from build123d import *

# Parameters (mm, degrees)
SKETCH3_R           = 1.25
BOSS_EXTRUDE1_DEPTH = 3
FILLET1_R           = 0.75
FILLET2_R           = 1


with BuildPart() as part:
    # Sketch3 → Boss-Extrude1 (new body)
    with BuildSketch(Plane(origin=(0, 0, 0), x_dir=(1, 0, 0), z_dir=(0, 1, 0))):
        with BuildLine():
            Line((-11.5, -24), (-11.5, -27))
            Line((-11.5, -27), (11.5, -27))
            Line((11.5, -27), (11.5, -24))
            Line((11.5, -24), (12.25, -24))
            ThreePointArc((12.25, -24), (15.25, -21), (12.25, -18))
            Line((12.25, -18), (11.5, -18))
            Line((11.5, -18), (11.5, -6))
            Line((11.5, -6), (12.25, -6))
            ThreePointArc((12.25, -6), (15.25, -3), (12.25, 0))
            Line((12.25, 0), (-12.25, 0))
            ThreePointArc((-12.25, 0), (-15.25, -3), (-12.25, -6))
            Line((-12.25, -6), (-11.5, -6))
            Line((-11.5, -6), (-11.5, -18))
            Line((-11.5, -18), (-12.25, -18))
            ThreePointArc((-12.25, -18), (-15.25, -21), (-12.25, -24))
            Line((-12.25, -24), (-11.5, -24))
        make_face()
        with Locations(Location((-12.25, -21, 0), (0, 0, 90))):
            Circle(SKETCH3_R, mode=Mode.SUBTRACT)
        with Locations(Location((-12.25, -3, 0), (0, 0, 90))):
            Circle(SKETCH3_R, mode=Mode.SUBTRACT)
        with Locations(Location((12.25, -3, 0), (0, 0, 270))):
            Circle(SKETCH3_R, mode=Mode.SUBTRACT)
        with Locations(Location((12.25, -21, 0), (0, 0, 270))):
            Circle(SKETCH3_R, mode=Mode.SUBTRACT)
    extrude(amount=BOSS_EXTRUDE1_DEPTH)

    # Fillet1
    fillet1_edges = [part.edges().sort_by_distance(p)[0] for p in [
        (-11.5, 1.5, 18),
        (-11.5, 1.5, 24),
        (-11.5, 1.5, 6),
        (11.5, 1.5, 6),
        (11.5, 1.5, 24),
        (11.5, 1.5, 18),
    ]]
    fillet(fillet1_edges, radius=FILLET1_R - 0.0001)  # a hair under: the kernel refuses the full size

    # Fillet2
    fillet2_edges = [part.edges().sort_by_distance(p)[0] for p in [
        (15.25, 3, 21),
        (15.25, 3, 3),
        (0, 3, 0),
        (-15.25, 3, 3),
        (-15.25, 3, 21),
        (-11.5, 3, 12),
        (-11.5, 3, 25.87495),
        (11.5, 3, 12),
        (-11.719640625, 3, 17.780359375),
        (-11.719640625, 3, 24.219640625),
        (-11.719640625, 3, 6.219640625),
        (11.719640625, 3, 6.219640625),
        (11.719640625, 3, 24.219640625),
        (11.719640625, 3, 17.780359375),
        (11.5, 3, 25.87495),
    ]]
    fillet(fillet2_edges, radius=FILLET2_R)


solid = part.part
Part model, mm, in its own coordinate system. A direction names the side the tool comes from. Give positions to 0.01 mm unless a question says otherwise; leave off trailing zeros. Order: outer loops, then holes, each group sorted by start corner. A loop starts at its lowest first (then second) coordinate and runs counter-clockwise, first axis right, second up. Notation, with made-up numbers: (40.25, 67) -> (76.25, 67) arc R6 cw to (76.25, 73) -> close; hole circle Ø10 at (18.5, 32.5). An arc over 180 degrees is marked (long way). Use one line per item in the form item = value.
(1) Saw through at A-A (z = 3). Write the cut outline in (x, y).
Solution:
outline = (-15.25, 0) -> (-13.5, 0) -> (-13.5, 3) -> (-14.25, 3) arc R1 ccw to (-15.25, 2) -> close; (-11, 0) -> (11, 0) -> (11, 3) -> (-11, 3) -> close; (13.5, 0) -> (15.25, 0) -> (15.25, 2) arc R1 ccw to (14.25, 3) -> (13.5, 3) -> close
(2) Pull direction Z, two halves, no side cores. Call faces 4 (the face through (13, 1, 22)), 5 (the face through (11.5, 1, 26)), 6 (the face through (0, 1, 27)), 7 (the face through (11.5, 1, 12)): +Z half, -Z half, draft (parallel to the pull), parting line (faces both ways), or undercut.
Solution:
face_4 = undercut
face_5 = draft
face_6 = +Z half
face_7 = undercut
(3) Tool access for faces 1 (the face through (11.199, 2.715, 25.859)), 2 (the face through (15.25, 0.99, 3.07)), 3 (the face through (-11.199, 2.715, 25.891)): list every direction of +Z, -Z, +X, -X, +Y, -Y with a clear straight run to the whole face (end or side of a thin tool).
Solution:
face_1 = +Z, +X, +Y
face_2 = +X, +Y, -Y
face_3 = +Z, -X, +Y
(4) Flat gauge pins, fed straight in: P1, Ø1.6, axis at y = 0.5, z = 13.5, coming from the +X side; P2, Ø1.5, axis at x = 1, z = 17, coming from the -Y side; P3, Ø1, axis at y = 1, z = 26, coming from the -X side; P4, Ø1.5, axis at x = -12.25, z = 3, coming from the -Y side. Where does each tip first touch, or does it go through?
Solution:
P1 = 11.5
P2 = 0
P3 = -11.5
P4 = through
(5) Saw through at B-B (y = 1.5). Count the separate pieces of the cut face and the enclosed holes in it, then the cut area to 3 significant figures.
Solution:
separate_pieces = 1
enclosed_holes = 4
area = 677 mm²
(6) Drill centre lines: line 1 (Z direction, x = -12.25, y = 1.1); line 2 (X direction, y = 2.1, z = 21); line 3 (X direction, y = 1.4, z = 3.5). Where is each one in solid material? Low to high. Write a range as from..to.
Solution:
line_1 = 0..1.75, 4.25..6, 18..19.75, 22.25..24
line_2 = -15.24..-13.5, -11..11, 13.5..15.24
line_3 = -15.21..-13.4, -11.1..11.1, 13.4..15.21
